Can you work these out from the model? Positions are in its coordinate system, mm. A direction names the side the tool comes from. Round coordinates to 2 decimals unless told otherwise and drop trailing zeros. Write each loop counter-clockwise with the first axis right and the second up, starting at its lowest first coordinate (ties: lowest second). Pieces come first, ordered by that corner, then holes. Notation, with made-up numbers: M 3.5,1.25 L 21.5,1.25 A15 ccw 21.5,13.25 Z; hole C -24.5,36 d8. An arc over 180 degrees is marked long. Answer as a JSON object with one key per item and string values. Group by question number.
1) If we mould it in two halves opening along Y, with no side actions, what happens to faces 1 (the flat face through (16, 0, 7)), 2 (the cylindrical face through (-5, 1, 6)), 3 (the cylindrical face through (19.947, -17.844, 7.395))? For each: +Y half, -Y half, draft (parallel to the pull), parting line (faces both ways), or undercut.
2) Please list where these lines run through material, in increasing order: L1, parallel to X at y = 1.5, z = 7.5; L2, parallel to Y at x = 14.5, z = 6.75; L3, parallel to Z at x = -5, y = 1.55. Write a range as [from, to].
3) Suppose I cut it at B-B, the plane x = -5. Write out the boundary of the cut face in (y, z), and give its area (3 significant figures).
4) Suppose I cut it at A-A, the plane z = 7.5. Write out the boundary of the cut face in (x, y), and give its area (3 significant figures).
5) Suppose I cut it at C-C, the plane y = -7.75. Write out the boundary of the cut face in (x, z), and give its area (3 significant figures).
6) On a 3-axis mill with a long thin cutter (end or side, diameter ignored), from which of +Z, -Z, +X, -X, +Y, -Y can I reach the whole of each face in a straight line? I mean faces 4 (the flat face through (2, -8, 7)), 5 (the flat face through (43.1, 0, 5.7)), 6 (the flat face through (0, -9, 7)). Say none if no direction works.
7) I'm going to push flat-ended pins straight in: pin 1 Ø7 at (y, z) = (-12, 10.5) entering from -X; pin 2 Ø4.5 at (x, z) = (42.5, 5) entering from -Y; pin 3 Ø1 at (y, z) = (-12, 9) entering from +X; pin 4 Ø2.5 at (x, z) = (43.16, 7.5) entering from -Y. Where does each tip first touch, or does it pass through?
Autodesk Inventor part; units mm, degrees
ref_plane "YZ Plane" through (0, 0, 0) normal (1, 0, 0) x (0, 1, 0)
ref_plane "XZ Plane" through (0, 0, 0) normal (0, 1, 0) x (-1, 0, 0)
ref_plane "XY Plane" through (0, 0, 0) normal (0, 0, 1) x (1, 0, 0)
sketch "Sketch1" plane through (0, 0, 0) normal (0, 0, 1) x (1, 0, 0)
  line L0 (0, -2) -> (0, -16)
  line L1 (2, -18) -> (19.1716, -18)
  line L2 (2, -2) -> (2, -14)
  line L3 (4, -16) -> (17.1716, -16)
  line L4 (20.5858, -17.4142) -> (37.4142, -0.5858)
  line L5 (18.5858, -15.4142) -> (30.5858, -3.4142)
  arc A0 (2, -14) -> (4, -16) centre (4, -14) ccw
  arc A1 (0, -16) -> (2, -18) centre (2, -16) ccw
  arc A2 (19.1716, -18) -> (20.5858, -17.4142) centre (19.1716, -16) ccw
  arc A3 (17.1716, -16) -> (18.5858, -15.4142) centre (17.1716, -14) ccw
  arc A4 (30.5858, -3.4142) -> (29.1716, 0) centre (29.1716, -2) ccw
  arc A5 (38.8284, 0) -> (37.4142, -0.5858) centre (38.8284, -2) ccw
  line L6 (2, -2) -> (2, -2)
  line L7 (-2, 0) -> (-10, 0)
  arc A6 (0, -2) -> (-2, 0) centre (-2, -2) ccw
  line L8 (-10, 0) -> (-10, 2)
  line L9 (-10, 2) -> (47.5, 2)
  line L10 (47.5, 2) -> (47.5, 0)
  arc A7 (4, 0) -> (2, -2) centre (4, -2) ccw
  line L11 (-10, 0) -> (-2, 0)
  line L12 (4, 0) -> (29.1716, 0)
  line L13 (38.8284, 0) -> (47.5, 0)
  line L14 (4, 0) -> (29.1716, 0)
  line L15 (38.8284, 0) -> (47.5, 0)
  line L16 (38.8284, 0) -> (38.8284, 2)
  point P0 (0, 0)
  point P1 (0, 0)
  point P2 (0, -18)
  point P3 (20, -18)
  point P4 (22, -16)
  point P5 (38, 0)
  point P6 (34, 0)
  point P7 (34, 0)
  dimension "d0" = 18
  dimension "d1" = 20
  dimension "d2" = 2
  dimension "d3" = 2
  dimension "d4" = 2
  dimension "d5" = 2
  dimension "d6" = 10
  dimension "d7" = 2
  dimension "d8" = 2
  dimension "d9" = 2
extrude "Extrusion1" add sketch "Sketch1" along normal blind 15
sketch "Sketch2" plane through (38.8284, 0, 0) normal (0, -1, 0) x (1, 0, 0)
  line L0 (8.6716, 0) -> (-48.8284, 0)
  line L1 (-48.8284, 0) -> (-48.8284, 5)
  line L2 (-48.8284, 0) -> (-48.8284, 15)
  line L3 (-48.8284, 5) -> (-48.8284, 0)
  line L4 (8.6716, 15) -> (-48.8284, 15)
  line L5 (-48.8284, 0) -> (-48.8284, 15)
  line L6 (-48.8284, 15) -> (-48.8284, 7.5)
  line L7 (-48.8284, 0) -> (-48.8284, 15)
  line L8 (-40.8284, 15) -> (-38.8284, 15)
  line L9 (-48.8284, 15) -> (-38.8284, 15)
  line L10 (-38.8284, 15) -> (-43.8284, 15)
  line L11 (-43.8284, 15) -> (-43.8284, 7.5)
  line L12 (-48.8284, 15) -> (-40.8284, 15)
  circle A0 centre (-43.8284, 7.5) radius 1.5
  line L13 (-18.2426, 15) -> (-1.4142, 15)
  line L14 (8.6716, 15) -> (-1.4142, 15)
  line L15 (-1.4142, 15) -> (4.3358, 15)
  line L16 (0, 15) -> (8.6716, 15)
  line L17 (4.3358, 15) -> (4.3358, 7.5)
  circle A1 centre (4.3358, 7.5) radius 1.5
  line L18 (8.6716, 0) -> (8.6716, 15)
  line L19 (8.6716, 15) -> (-48.8284, 15)
  line L20 (-48.8284, 15) -> (-48.8284, 0)
  line L21 (-48.8284, 0) -> (8.6716, 0)
  line L22 (8.6716, 0) -> (8.6716, 15)
  point P0 (-38.8284, 0)
  dimension "d12" = 5
  dimension "d13" = 5
  dimension "d19" = 3
  dimension "d20" = 3
extrude "Extrusion2" cut sketch "Sketch2" against normal up to surface (2 mm away) contours A1 | A0
sketch "Sketch3" plane through (-10, 2, 0) normal (0, 1, 0) x (1, 0, 0)
  line L0 (57.5, -15) -> (0, -15)
  line L1 (57.5, 0) -> (0, 0)
  line L2 (0, -15) -> (0, 0)
  line L3 (0, 0) -> (0, -15)
  line L4 (0, -15) -> (0, -7.5)
  line L5 (0, -7.5) -> (3.5, -7.5)
  circle A0 centre (5, -7.5) radius 1.5
  line L6 (5, -7.5) -> (3.5, -7.5)
  circle A1 centre (53.1642, -7.5) radius 1.5
  line L7 (53.1642, -6) -> (53.1642, -7.5)
  line L8 (53.1642, -7.5) -> (5, -7.5)
  line L9 (57.5, 0) -> (57.5, -15)
  point P0 (10, 0)
  dimension "d23" = 57.5
  dimension "d24" = 4.3358
properties part number "Motor_shroud"
Results:
{
 "1": {"face 1": "undercut", "face 2": "draft", "face 3": "-Y half"},
 "2": {"L1": "[-10, -6.5], [-3.5, 41.66], [44.66, 47.5]", "L2": "[-18, -16], [0, 2]", "L3": "[0, 6], [9, 15]"},
 "3": {"outline": "M 0,0 L 2,0 L 2,6 L 0,6 Z; M 0,9 L 2,9 L 2,15 L 0,15 Z", "area": "24.0 mm^2"},
 "4": {"outline": "M -10,0 L -6.5,0 L -6.5,2 L -10,2 Z; M -3.5,0 L -2,0 A2 cw 0,-2 L 0,-16 A2 ccw 2,-18 L 19.17,-18 A2 ccw 20.59,-17.41 L 37.41,-0.59 A2 cw 38.83,0 L 41.66,0 L 41.66,2 L -3.5,2 Z; M 44.66,0 L 47.5,0 L 47.5,2 L 44.66,2 Z; hole M 2,-14 A2 ccw 4,-16 L 17.17,-16 A2 ccw 18.59,-15.41 L 30.59,-3.41 A2 ccw 29.17,0 L 4,0 A2 ccw 2,-2 Z", "area": "248 mm^2"},
 "5": {"outline": "M 0,0 L 2,0 L 2,15 L 0,15 Z; M 26.25,0 L 30.25,0 L 30.25,15 L 26.25,15 Z", "area": "90.0 mm^2"},
 "6": {"face 4": "+Z, -Z", "face 5": "+Z, -Z, +X, -Y", "face 6": "+Z, -Z, -X, -Y"},
 "7": {"pin 1": "x = 0", "pin 2": "y = 0", "pin 3": "x = 26.5", "pin 4": "through"}
}
